Geometry: final body of the model. Coordinates: model frame, mm. Face numbers are marked on the shaded views. Coordinates: 2 decimals unless noted, no trailing zeros. Write each loop counter-clockwise with the first axis right and the second up, starting at its lowest first coordinate (ties: lowest second). Pieces come first, ordered by that corner, then holes. Notation, with made-up numbers: (69, 4.5) -> (82, 4.5) arc R34 ccw to (82, 40.5) -> close; hole circle Ø5 at (-28, -8). An arc over 180 degrees is marked (long way). One line per item, written item: value.
```python
from build123d import *

# Parameters (mm, degrees)
EXTRUDE_1_DEPTH                   = 7.5
HOLE_WIZARD_M12_1_D               = 10.2
HOLE_WIZARD_M12_1_DEPTH           = 29.25
HOLE_WIZARD_M12_1_TIP             = 3.064389157
HOLE_WIZARD_M12_1_ON_FACE_2_D     = 10.2
HOLE_WIZARD_M12_1_ON_FACE_2_DEPTH = 29.25
HOLE_WIZARD_M12_1_ON_FACE_2_TIP   = 3.064389157


with BuildPart() as part:
    # 草图1 → 凸台-拉伸1 (new body)
    with BuildSketch(Plane(origin=(0, 0, 0), x_dir=(1, 0, 0), z_dir=(0, 1, 0))):
        Polygon((2.986206823, -9.954022745), (10.113539979, -2.390880402), (7.127333155, 7.563142343), (-2.986206823, 9.954022745), (-10.113539979, 2.390880402), (-7.127333155, -7.563142343), align=None)
    extrude(amount=EXTRUDE_1_DEPTH)

    # M12 螺纹孔1
    with Locations(Plane(origin=(0, 0, 0), x_dir=(0, 0, -1), z_dir=(0, -1, 0))):
        with Locations((0, 0)):
            Hole(HOLE_WIZARD_M12_1_D / 2, depth=HOLE_WIZARD_M12_1_DEPTH)
            with Locations((0, 0, -(HOLE_WIZARD_M12_1_DEPTH + HOLE_WIZARD_M12_1_TIP / 2))):  # 118° drill point
                Cone(0, HOLE_WIZARD_M12_1_D / 2, HOLE_WIZARD_M12_1_TIP, mode=Mode.SUBTRACT)

    # M12 螺纹孔1 on face 2
    with Locations(Plane.ZX.offset(7.5)):
        with Locations((0, 0)):
            Hole(HOLE_WIZARD_M12_1_ON_FACE_2_D / 2, depth=HOLE_WIZARD_M12_1_ON_FACE_2_DEPTH)
            with Locations((0, 0, -(HOLE_WIZARD_M12_1_ON_FACE_2_DEPTH + HOLE_WIZARD_M12_1_ON_FACE_2_TIP / 2))):  # 118° drill point
                Cone(0, HOLE_WIZARD_M12_1_ON_FACE_2_D / 2, HOLE_WIZARD_M12_1_ON_FACE_2_TIP, mode=Mode.SUBTRACT)


solid = part.part
```
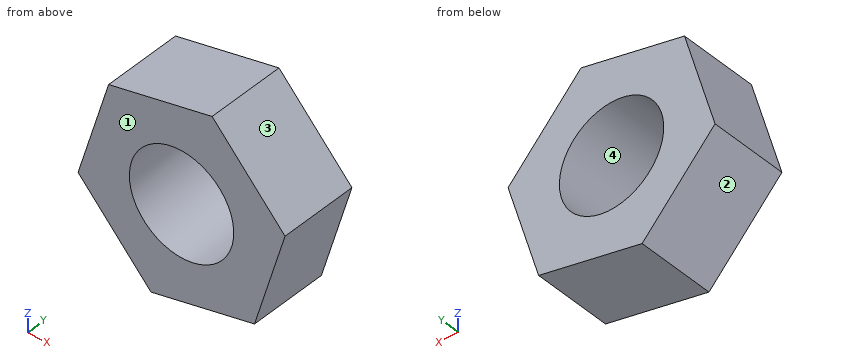
(1) Section C-C (z = 0). Return the cut outline in (x, y).
Responses:
outline: (-9.4, 0) -> (-5.1, 0) -> (-5.1, 7.5) -> (-9.4, 7.5) -> close; (5.1, 0) -> (9.4, 0) -> (9.4, 7.5) -> (5.1, 7.5) -> close
(2) First-contact query: pin 1 (1 mm diameter, centred on x = -4.5, z = 0, fed in from -Y); pin 2 (2 mm diameter, centred on y = 3.5, z = -3.5, fed in from -X); pin 3 (3 mm diameter, centred on y = 6, z = 6.5, fed in from +X). Flat tips, straight axial feed; report the tip coordinate or a pass-through.
Responses:
pin 1: passes through
pin 2: stops at x = -10.01
pin 3: stops at x = 7.65
(3) Pull-direction query (Z, two-part tool) for the marked faces 1, 2, 3 and 4; classes: released by +Z, released by -Z, zero draft, split by the parting line, or undercut.
Responses:
face 1: zero draft
face 2: released by -Z
face 3: released by +Z
face 4: undercut
(4) Section A-A (x = 0). Return the cut outline in (y, z).
Responses:
outline: (0, -9.25) -> (7.5, -9.25) -> (7.5, -5.1) -> (0, -5.1) -> close; (0, 5.1) -> (7.5, 5.1) -> (7.5, 9.25) -> (0, 9.25) -> close
(5) Line query: line 1 (Z direction, x = 0, y = 4); line 2 (X direction, y = 2.5, z = 2.75); line 3 (X direction, y = 4, z = 0). Output: solid intervals per line, ascending. Write a range as [from, to].
Responses:
line 1: z = [-9.25, -5.1], [5.1, 9.25]
line 2: x = [-8.57, -4.3], [4.3, 9.78]
line 3: x = [-9.4, -5.1], [5.1, 9.4]
(6) Section B-B (y = 6.25). Return the cut outline in (x, z).
Responses:
outline: (-10.11, -2.39) -> (-2.99, -9.95) -> (7.13, -7.56) -> (10.11, 2.39) -> (2.99, 9.95) -> (-7.13, 7.56) -> close; hole circle Ø10.2 at (0, 0)
(7) Section D-D (z = -8). Return the cut outline in (x, y).
Responses:
outline: (-4.83, 0) -> (5.28, 0) -> (5.28, 7.5) -> (-4.83, 7.5) -> close
